Can you work these out from the model? Positions are in its coordinate system, mm. Give positions to 0.01 mm unless a question says otherwise; leave off trailing zeros. Loops run counter-clockwise (first coordinate to the right, second up) from the corner with the lowest first, then second, coordinate; pieces in that order, holes last. Notation, with made-up numbers: (-7, 1) - (14, 1) arc R29 ccw to (14, 22) - close; hole circle Ø7 at (89.5, 57.25). An arc over 180 degrees is marked (long way). Answer as a JSON object with one key per item and string values. Group by question number.
Item 1: Suppose I cut it at A-A on y = -29.5. Write out the boundary of the cut face in (x, z), and give its area (3 significant figures).
Item 2: Please list where these lines run through material, in increasing order: L1, parallel to Z at x = -18.5, y = -44.5; L2, parallel to Y at x = -13, z = -8.25; L3, parallel to X at y = -10.5, z = -4.5.
Item 3: Thinking about a two-plate mould opening in Z: for faces 1 (the flat face through (-12, -10, -10)), 2 (the cylindrical face through (-39.96, -1.76, -0.07)), 3 (the cylindrical face through (47.69, 15.02, -7.46)), which applies, pulls with the +Z half, pulls with the -Z half, needs draft (parallel to the pull), parting line crosses it, or undercut?
Item 4: Will these pins go through, and if not, where does the flat tip stop? pin 1 (3 mm diameter, centred on y = -18.5, z = -2, fed in from -X); pin 2 (6 mm diameter, centred on x = 40, z = -1, fed in from -Y); pin 3 (12 mm diameter, centred on y = -37.5, z = -8, fed in from +X).
Item 5: Suppose I cut it at B-B on x = -37. Write out the boundary of the cut face in (y, z).
from build123d import *

# Parameters (mm, degrees)
SKETCH1_R           = 50
BOSS_EXTRUDE1_DEPTH = 10
SKETCH2_W           = 10
SKETCH2_H           = 10


with BuildPart() as part:
    # Sketch1 → Boss-Extrude1 (new, symmetric)
    with BuildSketch(Plane.XY):
        Circle(SKETCH1_R)
        with BuildLine():
            Line((-1, 14.966629547), (-0.5, 12.489995997))
            ThreePointArc((-0.5, 12.489995997), (0, 12.5), (0.5, 12.489995997))
            Line((0.5, 12.489995997), (1, 14.966629547))
            ThreePointArc((1, 14.966629547), (2.346516976, 14.815325109), (3.673886362, 14.543127552))
            Line((3.673886362, 14.543127552), (3.384092765, 12.033200578))
            ThreePointArc((3.384092765, 12.033200578), (3.86271243, 11.888206454), (4.335149281, 11.724183584))
            Line((4.335149281, 11.724183584), (5.575999395, 13.925093563))
            ThreePointArc((5.575999395, 13.925093563), (6.809857496, 13.365097863), (7.98814713, 12.696042904))
            Line((7.98814713, 12.696042904), (6.936926951, 10.398511647))
            ThreePointArc((6.936926951, 10.398511647), (7.347315654, 10.11271243), (7.745943945, 9.810726395))
            Line((7.745943945, 9.810726395), (9.606181119, 11.5204724))
            ThreePointArc((9.606181119, 11.5204724), (10.606601718, 10.606601718), (11.5204724, 9.606181119))
            Line((11.5204724, 9.606181119), (9.810726395, 7.745943945))
            ThreePointArc((9.810726395, 7.745943945), (10.11271243, 7.347315654), (10.398511647, 6.936926951))
            Line((10.398511647, 6.936926951), (12.696042904, 7.98814713))
            ThreePointArc((12.696042904, 7.98814713), (13.365097863, 6.809857496), (13.925093563, 5.575999395))
            Line((13.925093563, 5.575999395), (11.724183584, 4.335149281))
            ThreePointArc((11.724183584, 4.335149281), (11.888206454, 3.86271243), (12.033200578, 3.384092765))
            Line((12.033200578, 3.384092765), (14.543127552, 3.673886362))
            ThreePointArc((14.543127552, 3.673886362), (14.815325109, 2.346516976), (14.966629547, 1))
            Line((14.966629547, 1), (12.489995997, 0.5))
            ThreePointArc((12.489995997, 0.5), (12.5, 0), (12.489995997, -0.5))
            Line((12.489995997, -0.5), (14.966629547, -1))
            ThreePointArc((14.966629547, -1), (14.815325109, -2.346516976), (14.543127552, -3.673886362))
            Line((14.543127552, -3.673886362), (12.033200578, -3.384092765))
            ThreePointArc((12.033200578, -3.384092765), (11.888206454, -3.86271243), (11.724183584, -4.335149281))
            Line((11.724183584, -4.335149281), (13.925093563, -5.575999395))
            ThreePointArc((13.925093563, -5.575999395), (13.365097863, -6.809857496), (12.696042904, -7.98814713))
            Line((12.696042904, -7.98814713), (10.398511647, -6.936926951))
            ThreePointArc((10.398511647, -6.936926951), (10.11271243, -7.347315654), (9.810726395, -7.745943945))
            Line((9.810726395, -7.745943945), (11.5204724, -9.606181119))
            ThreePointArc((11.5204724, -9.606181119), (10.606601718, -10.606601718), (9.606181119, -11.5204724))
            Line((9.606181119, -11.5204724), (7.745943945, -9.810726395))
            ThreePointArc((7.745943945, -9.810726395), (7.347315654, -10.11271243), (6.936926951, -10.398511647))
            Line((6.936926951, -10.398511647), (7.98814713, -12.696042904))
            ThreePointArc((7.98814713, -12.696042904), (6.809857496, -13.365097863), (5.575999395, -13.925093563))
            Line((5.575999395, -13.925093563), (4.335149281, -11.724183584))
            ThreePointArc((4.335149281, -11.724183584), (3.86271243, -11.888206454), (3.384092765, -12.033200578))
            Line((3.384092765, -12.033200578), (3.673886362, -14.543127552))
            ThreePointArc((3.673886362, -14.543127552), (2.346516976, -14.815325109), (1, -14.966629547))
            Line((1, -14.966629547), (0.5, -12.489995997))
            ThreePointArc((0.5, -12.489995997), (0, -12.5), (-0.5, -12.489995997))
            Line((-0.5, -12.489995997), (-1, -14.966629547))
            ThreePointArc((-1, -14.966629547), (-2.346516976, -14.815325109), (-3.673886362, -14.543127552))
            Line((-3.673886362, -14.543127552), (-3.384092765, -12.033200578))
            ThreePointArc((-3.384092765, -12.033200578), (-3.86271243, -11.888206454), (-4.335149281, -11.724183584))
            Line((-4.335149281, -11.724183584), (-5.575999395, -13.925093563))
            ThreePointArc((-5.575999395, -13.925093563), (-6.809857496, -13.365097863), (-7.98814713, -12.696042904))
            Line((-7.98814713, -12.696042904), (-6.936926951, -10.398511647))
            ThreePointArc((-6.936926951, -10.398511647), (-7.347315654, -10.11271243), (-7.745943945, -9.810726395))
            Line((-7.745943945, -9.810726395), (-9.606181119, -11.5204724))
            ThreePointArc((-9.606181119, -11.5204724), (-10.606601718, -10.606601718), (-11.5204724, -9.606181119))
            Line((-11.5204724, -9.606181119), (-9.810726395, -7.745943945))
            ThreePointArc((-9.810726395, -7.745943945), (-10.11271243, -7.347315654), (-10.398511647, -6.936926951))
            Line((-10.398511647, -6.936926951), (-12.696042904, -7.98814713))
            ThreePointArc((-12.696042904, -7.98814713), (-13.365097863, -6.809857496), (-13.925093563, -5.575999395))
            Line((-13.925093563, -5.575999395), (-11.724183584, -4.335149281))
            ThreePointArc((-11.724183584, -4.335149281), (-11.888206454, -3.86271243), (-12.033200578, -3.384092765))
            Line((-12.033200578, -3.384092765), (-14.543127552, -3.673886362))
            ThreePointArc((-14.543127552, -3.673886362), (-14.815325109, -2.346516976), (-14.966629547, -1))
            Line((-14.966629547, -1), (-12.489995997, -0.5))
            ThreePointArc((-12.489995997, -0.5), (-12.5, 0), (-12.489995997, 0.5))
            Line((-12.489995997, 0.5), (-14.966629547, 1))
            ThreePointArc((-14.966629547, 1), (-14.815325109, 2.346516976), (-14.543127552, 3.673886362))
            Line((-14.543127552, 3.673886362), (-12.033200578, 3.384092765))
            ThreePointArc((-12.033200578, 3.384092765), (-11.888206454, 3.86271243), (-11.724183584, 4.335149281))
            Line((-11.724183584, 4.335149281), (-13.925093563, 5.575999395))
            ThreePointArc((-13.925093563, 5.575999395), (-13.365097863, 6.809857496), (-12.696042904, 7.98814713))
            Line((-12.696042904, 7.98814713), (-10.398511647, 6.936926951))
            ThreePointArc((-10.398511647, 6.936926951), (-10.11271243, 7.347315654), (-9.810726395, 7.745943945))
            Line((-9.810726395, 7.745943945), (-11.5204724, 9.606181119))
            ThreePointArc((-11.5204724, 9.606181119), (-10.606601718, 10.606601718), (-9.606181119, 11.5204724))
            Line((-9.606181119, 11.5204724), (-7.745943945, 9.810726395))
            ThreePointArc((-7.745943945, 9.810726395), (-7.347315654, 10.11271243), (-6.936926951, 10.398511647))
            Line((-6.936926951, 10.398511647), (-7.98814713, 12.696042904))
            ThreePointArc((-7.98814713, 12.696042904), (-6.809857496, 13.365097863), (-5.575999395, 13.925093563))
            Line((-5.575999395, 13.925093563), (-4.335149281, 11.724183584))
            ThreePointArc((-4.335149281, 11.724183584), (-3.86271243, 11.888206454), (-3.384092765, 12.033200578))
            Line((-3.384092765, 12.033200578), (-3.673886362, 14.543127552))
            ThreePointArc((-3.673886362, 14.543127552), (-2.346516976, 14.815325109), (-1, 14.966629547))
        make_face(mode=Mode.SUBTRACT)
    extrude(amount=BOSS_EXTRUDE1_DEPTH, both=True)

    # Sketch2 → Cut-Revolve1 (revolve, cut)
    with BuildSketch(Plane(origin=(0, 0, 0), x_dir=(0, 0, -1), z_dir=(1, 0, 0)), mode=Mode.PRIVATE) as cut_revolve1_sk:
        with Locations((0, 45)):
            Rectangle(SKETCH2_W, SKETCH2_H)
    revolve(cut_revolve1_sk.sketch.rotate(Axis((0, 0, 1000), (0, 0, -1)), 90), axis=Axis((0, 0, 1000), (0, 0, -1)), mode=Mode.SUBTRACT)


solid = part.part
Worked out:
{
 "1": {"outline": "(-40.37, -10) - (40.37, -10) - (40.37, -5) - (27.01, -5) - (27.01, 5) - (40.37, 5) - (40.37, 10) - (-40.37, 10) - (-40.37, 5) - (-27.01, 5) - (-27.01, -5) - (-40.37, -5) - close", "area": "1,350 mm2"},
 "2": {"L1": "z = -10 to -5, 5 to 10", "L2": "y = -48.28 to -7.48, -5.05 to -3.5, -0.6 to 0.6, 3.5 to 5.05, 7.48 to 48.28", "L3": "x = -38.6 to -10.71, -8.5 to -6.98, 6.98 to 8.5, 10.71 to 38.6"},
 "3": {"face 1": "pulls with the -Z half", "face 2": "undercut", "face 3": "needs draft"},
 "4": {"pin 1": "stops at x = -36.21", "pin 2": "stops at y = -15.2", "pin 3": "stops at x = 38.83"},
 "5": {"outline": "(-33.63, -10) - (33.63, -10) - (33.63, -5) - (15.2, -5) - (15.2, 5) - (33.63, 5) - (33.63, 10) - (-33.63, 10) - (-33.63, 5) - (-15.2, 5) - (-15.2, -5) - (-33.63, -5) - close"}
}
